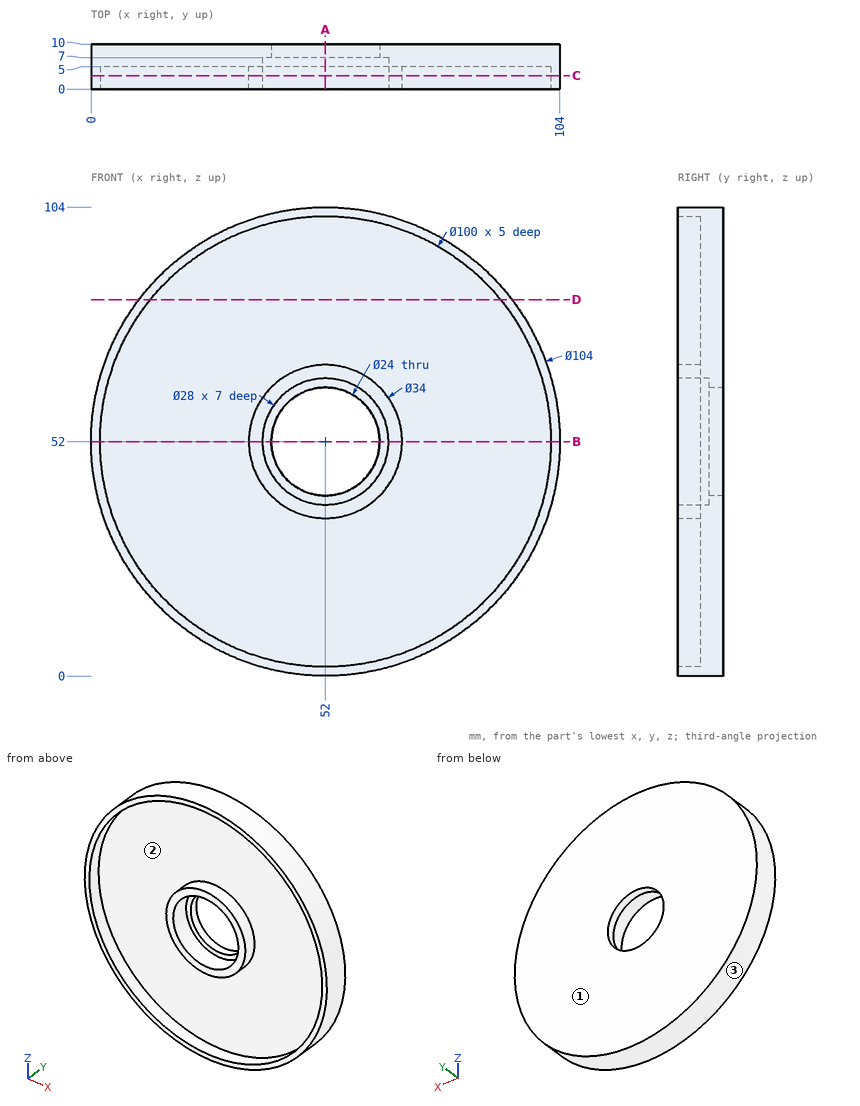
Verification items for this drawing (mm, ordinates from the low corner). Give positions to 0.01 mm unless a question says otherwise; leave off trailing zeros. Write each loop counter-clockwise with the first axis right and the second up, starting at its lowest first coordinate (ties: lowest second). Pieces come first, ordered by that corner, then holes. Notation, with made-up numbers: (-18, -31.5) -> (41, -31.5) arc R15 cw to (41, -13.5) -> close; hole circle Ø4 at (61.5, 42.25). An arc over 180 degrees is marked (long way). Write item = value, one per line.
Item 1: Sectioned sample at B-B on z = 52. Record the boundary of the cut face in (x, y), and give its area (3 significant figures).
Output:
outline = (0, 0) -> (2, 0) -> (2, 5) -> (35, 5) -> (35, 0) -> (38, 0) -> (38, 7) -> (40, 7) -> (40, 10) -> (0, 10) -> close; (64, 7) -> (66, 7) -> (66, 0) -> (69, 0) -> (69, 5) -> (102, 5) -> (102, 0) -> (104, 0) -> (104, 10) -> (64, 10) -> close
area = 442 mm^2
Item 2: Sectioned sample at A-A on x = 52. Record the boundary of the cut face in (y, z).
Output:
outline = (0, 0) -> (10, 0) -> (10, 40) -> (7, 40) -> (7, 38) -> (0, 38) -> (0, 35) -> (5, 35) -> (5, 2) -> (0, 2) -> close; (0, 66) -> (7, 66) -> (7, 64) -> (10, 64) -> (10, 104) -> (0, 104) -> (0, 102) -> (5, 102) -> (5, 69) -> (0, 69) -> close
Item 3: Sectioned sample at D-D on z = 83.5. Record the boundary of the cut face in (x, y).
Output:
outline = (10.63, 0) -> (13.17, 0) -> (13.17, 5) -> (90.83, 5) -> (90.83, 0) -> (93.37, 0) -> (93.37, 10) -> (10.63, 10) -> close
Item 4: Scan lines: probe 1 along X at (y, z) = (2.5, 52); probe 2 along Z at (x, y) = (37, 0.5); probe 3 along X at (y, z) = (1.5, 48). Record each from-to range of solid material in increasing order. Write a range as from..to.
Output:
probe_1 = 0..2, 35..38, 66..69, 102..104
probe_2 = 2.21..4.3, 44..60, 99.7..101.79
probe_3 = 0.15..2.16, 35.48..38.58, 65.42..68.52, 101.84..103.85
Item 5: Sectioned sample at C-C on y = 3. Record the boundary of the cut face in (x, z).
Output:
outline = circle Ø104 at (52, 52); circle Ø34 at (52, 52); hole circle Ø100 at (52, 52); hole circle Ø28 at (52, 52)
Item 6: Gauge pin test, flat ends, axial feed: pin 1 (1.5 mm diameter, centred on x = 82, y = 3, fed in from -Z); pin 2 (6 mm diameter, centred on x = 73, y = 7, fed in from -Z); pin 3 (4 mm diameter, centred on x = 20, z = 57, fed in from -Y). Record the tip position at first contact, or that the pin passes through.
Output:
pin_1 = 9.01
pin_2 = 3.21
pin_3 = 5
Item 7: Release check for a two-part mould opening along X. For the marked faces 1, 2 and 3 record: +X half, -X half, draft (parallel to the pull), parting line (faces both ways), or undercut.
Output:
face_1 = draft
face_2 = undercut
face_3 = parting line
